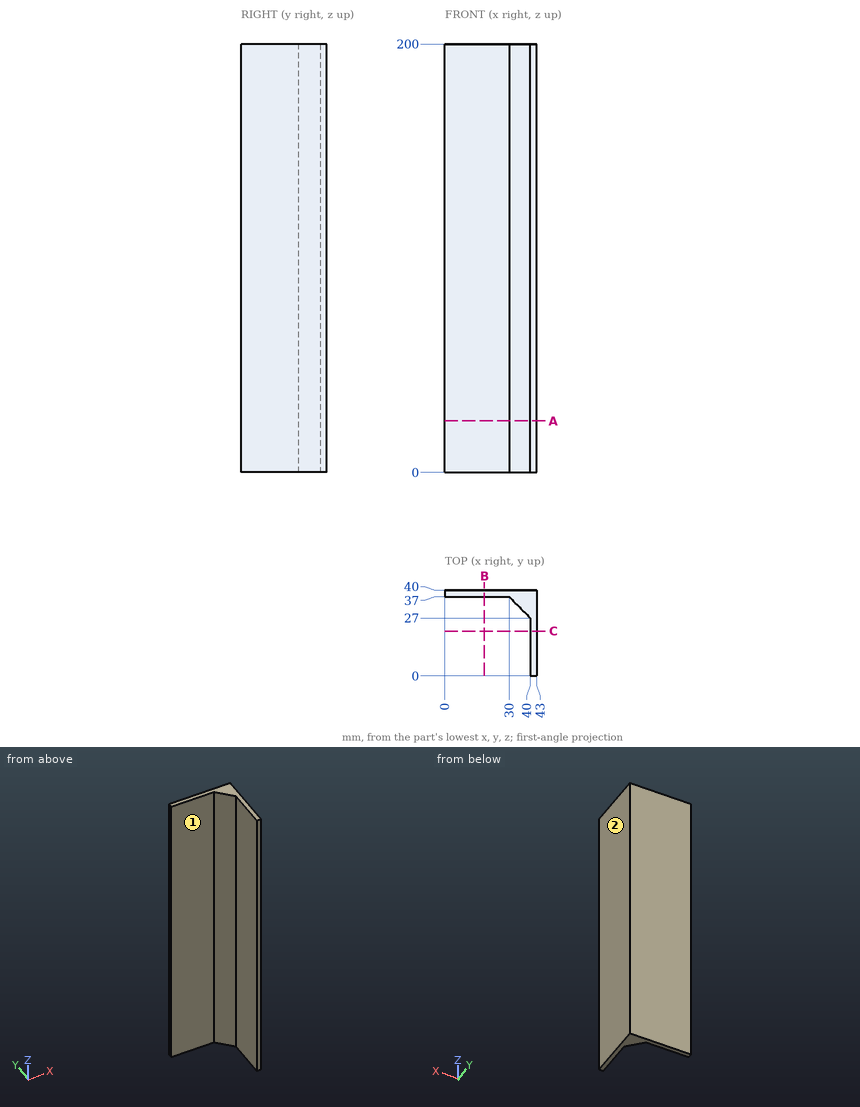
Geometry check sheet. Reference: drawing and pictorial views, mm from the part's lowest x, y, z. A direction names the side the tool comes from. Round coordinates to 2 decimals unless told otherwise and drop trailing zeros. Write each loop counter-clockwise with the first axis right and the second up, starting at its lowest first coordinate (ties: lowest second). Pieces come first, ordered by that corner, then holes.
(1) Depth check by flat-ended pin: pin 1 Ø1.5 at (y, z) = (11.5, 105.5) entering from -X; pin 2 Ø9 at (x, z) = (9, 128) entering from -Y; pin 3 Ø12 at (x, z) = (33.5, 137) entering from -Y. Enter the tip coordinate at first touch or a pass-through.
Returned:
pin 1: stops at x = 40
pin 2: stops at y = 37
pin 3: stops at y = 27.5
(2) Material ranges on line 1 (X direction, y = 24.5, z = 24.5); line 2 (Y direction, x = 9, z = 167.5); line 3 (X direction, y = 33, z = 39), recorded low to high.
Returned:
line 1: x = 40 to 43
line 2: y = 37 to 40
line 3: x = 34 to 43
(3) Section check B-B (x = 18.5). Enter the section's corners in (y, z).
Returned:
outline: (37, 0) - (40, 0) - (40, 200) - (37, 200) - close
(4) Access from +Z, -Z, +X, -X, +Y, -Y to the whole of each face (thin tool, end or side, straight path). Record for the marked faces 1 and 2.
Returned:
face 1: +Z, -Z, -X, -Y
face 2: +Z, -Z, +X, +Y, -Y
(5) Section check A-A (z = 24). Enter the section's corners in (x, y), plus the area to 3 significant figures.
Returned:
outline: (0, 37) - (30, 37) - (40, 27) - (40, 0) - (43, 0) - (43, 40) - (0, 40) - close
area: 290 mm2
(6) Section check C-C (y = 21). Enter the section's corners in (x, z).
Returned:
outline: (40, 0) - (43, 0) - (43, 200) - (40, 200) - close
